Read the model definition and answer for the solid it produces. Units are mm, in the model's axes. A direction names the side the tool comes from. Coordinates: 2 decimals unless noted, no trailing zeros. Write each loop counter-clockwise with the first axis right and the second up, starting at its lowest first coordinate (ties: lowest second). Pieces come first, ordered by that corner, then holes.
1) Which of the six approach directions +Z, -Z, +X, -X, +Y, -Y give full straight-line access (tool end or side, diameter ignored) to faces 4 (the face through (13, 14, 32)), 5 (the face through (21.6, 10.05, 15.99)), 6 (the face through (9.6, 17.05, 67.18))?
2) Find the intervals of material crossed by line 1 (X direction, y = 17, z = 16.45); line 2 (Y direction, x = 10.8, z = 67.2); line 3 (Z direction, x = 13, y = 9), in increasing order.
3) The part is cut by section D-D (x = 13). Determine the outline of the cut face in (y, z), then the cut area to 3 significant figures.
4) Each of these flat-tipped pins is pushed along its axis until it touches: pin 1 Ø1.9 at (x, y) = (10.8, 10) entering from -Z; pin 2 Ø6.5 at (x, z) = (14.5, 7.5) entering from +Y; pin 3 Ø8 at (x, z) = (22, 62) entering from -Y; pin 4 Ø4 at (x, y) = (22.8, 17) entering from -Z. Where does it stop, or does it pass through?
5) The part is cut by section B-B (y = 15). Determine the outline of the cut face in (x, z).
6) The part is cut by section A-A (x = 17). Determine the outline of the cut face in (y, z), then the cut area to 3 significant figures.
7) The part is cut by section C-C (z = 38). Determine the outline of the cut face in (x, y), then the cut area to 3 significant figures.
8) Determine the mould class of faces 1 (the face through (12, 10, 16)), 2 (the face through (16.86, 4.57, 17.6)), 3 (the face through (11, 14, 36)) for opening direction Y: +Y half, -Y half, draft (parallel to the pull), parting line (faces both ways), or undercut.
from build123d import *

# Parameters (mm, degrees)
SKETCH003_R                          = 1.2
EXTRUDE003_DEPTH                     = 6
EXTRUDE004_DEPTH                     = 5
SKETCH002_AS_DRAWN_W                 = 3
SKETCH002_AS_DRAWN_H                 = 17.571103
EXTRUDE002_DEPTH                     = 15
EXTRUDE002_ONTO_SKETCH002_ROLL_ANGLE = 90
SKETCH_R                             = 1.5
EXTRUDE_DEPTH                        = 36
SKETCH001_AS_DRAWN_R                 = 13.5
EXTRUDE001_DEPTH                     = 20
EXTRUDE001_ONTO_SKETCH001_ROLL_ANGLE = 90


with BuildPart() as mounting_holes_top:
    # Sketch003 → Extrude003 (new body)
    with BuildSketch(Plane.XY.offset(70)):
        with Locations((10.8, 17)):
            Circle(SKETCH003_R)
        with Locations((22.8, 17)):
            Circle(SKETCH003_R)
        with Locations((10.8, 10)):
            Circle(SKETCH003_R)
        with Locations((22.8, 10)):
            Circle(SKETCH003_R)
    extrude(amount=-EXTRUDE003_DEPTH)


with BuildPart() as fusion:
    # Sketch003 → Extrude004 (new body)
    with BuildSketch(Plane.XY.offset(70)):
        with Locations((10.8, 17)):
            Circle(SKETCH003_R)
        with Locations((22.8, 17)):
            Circle(SKETCH003_R)
        with Locations((10.8, 10)):
            Circle(SKETCH003_R)
        with Locations((22.8, 10)):
            Circle(SKETCH003_R)
    extrude(amount=EXTRUDE004_DEPTH)


with BuildPart() as fusion_1:
    # Extrude004 placement: moved
    add(fusion.part.moved(Location((0, 0, -57))))

    # Fusion: union Mounting_Holes_Top
    add(mounting_holes_top.part)


with BuildPart() as extrude002:
    # Sketch002 as drawn → Extrude002 (new)
    with BuildSketch(Plane.XY):
        with Locations((0, 38.493945)):
            Rectangle(SKETCH002_AS_DRAWN_W, SKETCH002_AS_DRAWN_H)
        Polygon((6, 38.708394), (6, 29.708394), (20, 29.708394), (20, 47.279497), align=None)
        Polygon((-6, 38.708394), (-6, 29.708394), (-20, 29.708394), (-20, 47.279497), align=None)
    extrude(amount=-EXTRUDE002_DEPTH)


with BuildPart() as extrude002_1:
    # Extrude002 onto Sketch002 roll: moved
    add(extrude002.part.rotate(Axis((0, 0, 0), (1, 0, 0)), EXTRUDE002_ONTO_SKETCH002_ROLL_ANGLE))


with BuildPart() as extrude002_2:
    # Extrude002 onto Sketch002 placement: moved
    add(extrude002_1.part.moved(Location((17, 0, 0))))


with BuildPart() as extrude002_3:
    # Extrude002 placement: moved
    add(extrude002_2.part.moved(Location((0, 5, 0))))


with BuildPart() as extrude_body:
    # Sketch → Extrude (new body)
    with BuildSketch(Plane.YZ):
        with Locations((12.5, 35)):
            Circle(SKETCH_R)
        with BuildLine():
            Line((4, 52), (4, 19))
            ThreePointArc((4, 19), (4.585786, 17.585786), (6, 17))
            Line((6, 17), (45, 17))
            Line((45, 17), (45, 32))
            Line((8, 32), (45, 32))
            Line((8, 52), (8, 32))
            ThreePointArc((8, 52), (6, 54), (4, 52))
        make_face()
        with BuildLine():
            Line((6, 15), (45, 15))
            Line((45, 15), (45, -5))
            Line((45, -5), (6, -5))
            ThreePointArc((4, -3), (4.585786, -4.414214), (6, -5))
            Line((4, -3), (4, 13))
            ThreePointArc((6, 15), (4.585786, 14.414214), (4, 13))
        make_face()
    extrude(amount=EXTRUDE_DEPTH)


with BuildPart() as extrude_body_1:
    # Extrude placement: moved
    add(extrude_body.part.moved(Location((-1, 0, 0))))


with BuildPart() as cut002:
    # Sketch001 as drawn → Extrude001 (new)
    with BuildSketch(Plane.XY):
        with BuildLine():
            Line((-10, 70), (10, 70))
            Line((10, 70), (10, 64.842719))
            ThreePointArc((10, 41.157281), (15.5, 53), (10, 64.842719))
            Line((10, 41.157281), (10, 7))
            ThreePointArc((3, 0), (7.949747, 2.050253), (10, 7))
            Line((-3, 0), (3, 0))
            ThreePointArc((-10, 7), (-7.949747, 2.050253), (-3, 0))
            Line((-10, 41.157281), (-10, 7))
            ThreePointArc((-10, 64.842719), (-15.5, 53), (-10, 41.157281))
            Line((-10, 70), (-10, 64.842719))
        make_face()
        with Locations((0, 53)):
            Circle(SKETCH001_AS_DRAWN_R, mode=Mode.SUBTRACT)
    extrude(amount=-EXTRUDE001_DEPTH)


with BuildPart() as cut002_1:
    # Extrude001 onto Sketch001 roll: moved
    add(cut002.part.rotate(Axis((0, 0, 0), (1, 0, 0)), EXTRUDE001_ONTO_SKETCH001_ROLL_ANGLE))


with BuildPart() as cut002_2:
    # Extrude001 onto Sketch001 placement: moved
    add(cut002_1.part.moved(Location((17, 0, 0))))

    # Cut: cut Extrude body
    add(extrude_body_1.part, mode=Mode.SUBTRACT)

    # Cut001: cut Extrude002
    add(extrude002_3.part, mode=Mode.SUBTRACT)

    # Cut002: cut Fusion
    add(fusion_1.part, mode=Mode.SUBTRACT)


solid = cut002_2.part
Reported:
1. face 4: +X, -X, +Y
1. face 5: -Z
1. face 6: +Z
2. line 1: x = 7 to 9.6, 12 to 21.6, 24 to 27
2. line 2: y = 0 to 8.8, 11.2 to 15.8, 18.2 to 20
2. line 3: z = 15 to 17, 32 to 40.11, 65.89 to 70
3. outline: (0, 0.07) - (4, 0.07) - (4, 13) arc R2 cw to (6, 15) - (20, 15) - (20, 17) - (6, 17) arc R2 cw to (4, 19) - (4, 40.11) - (0, 40.11) - close; (0, 65.89) - (20, 65.89) - (20, 70) - (0, 70) - close; (8, 32) - (20, 32) - (20, 40.11) - (8, 40.11) - close; hole circle Ø3 at (12.5, 35)
3. area: 366 mm2
4. pin 1: stops at z = 32
4. pin 2: stops at y = 4
4. pin 3: stops at y = 0
4. pin 4: stops at z = 15
5. outline: (7, 15) - (27, 15) - (27, 17) - (7, 17) - close; (7, 41.16) - (11, 38.71) - (11, 32) - (15.5, 32) - (15.5, 39.58) arc R13.5 cw (long way) to (18.5, 39.58) - (18.5, 32) - (23, 32) - (23, 38.71) - (27, 41.16) arc R15.5 ccw to (27, 64.84) - (27, 70) - (7, 70) - (7, 64.84) arc R15.5 ccw to start
6. outline: (0, 0) - (4, 0) - (4, 13) arc R2 cw to (6, 15) - (20, 15) - (20, 17) - (6, 17) arc R2 cw to (4, 19) - (4, 39.5) - (0, 39.5) - close; (0, 66.5) - (20, 66.5) - (20, 70) - (0, 70) - close
6. area: 262 mm2
7. outline: (7, 0) - (27, 0) - (27, 4) - (7, 4) - close; (11, 8) - (15.5, 8) - (15.5, 20) - (11, 20) - close; (18.5, 8) - (23, 8) - (23, 20) - (18.5, 20) - close
7. area: 188 mm2
8. face 1: undercut
8. face 2: +Y half
8. face 3: draft
